The figure shows three views and two pictorial views of one solid part (mm, origin at its lowest corner). Answer the questions. Coordinates: 2 decimals unless noted, no trailing zeros. Order: outer loops, then holes, each group sorted by start corner. A loop starts at its lowest first (then second) coordinate and runs counter-clockwise, first axis right, second up. Notation, with made-up numbers: (-3.5, 69) -> (38.5, 69) arc R24 ccw to (38.5, 87) -> close; hole circle Ø4 at (-25.5, -30.5). An arc over 180 degrees is marked (long way). Write item = value, one per line.
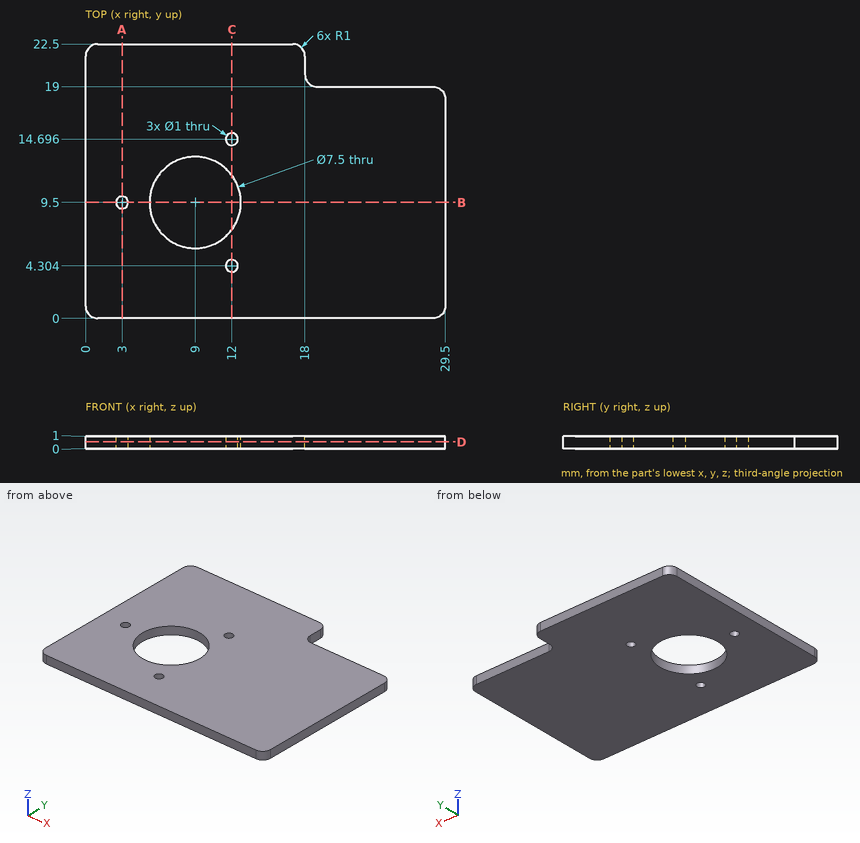
Q1. Section B-B, the plane y = 9.5 is taken. Give the vertices of the cut face in (x, z), plus the area to 3 significant figures.
The answers:
outline = (0, 0) -> (2.5, 0) -> (2.5, 1) -> (0, 1) -> close; (3.5, 0) -> (5.25, 0) -> (5.25, 1) -> (3.5, 1) -> close; (12.75, 0) -> (29.5, 0) -> (29.5, 1) -> (12.75, 1) -> close
area = 21.0 mm2
Q2. Section D-D, the plane z = 0.55 is taken. Give the vertices of the cut face in (x, y).
The answers:
outline = (0, 1) arc R1 ccw to (1, 0) -> (28.5, 0) arc R1 ccw to (29.5, 1) -> (29.5, 18) arc R1 ccw to (28.5, 19) -> (19, 19) arc R1 cw to (18, 20) -> (18, 21.5) arc R1 ccw to (17, 22.5) -> (1, 22.5) arc R1 ccw to (0, 21.5) -> close; hole circle Ø1 at (3, 9.5); hole circle Ø7.5 at (9, 9.5); hole circle Ø1 at (12, 4.3); hole circle Ø1 at (12, 14.7)
Q3. Section C-C, the plane x = 12 is taken. Give the vertices of the cut face in (y, z).
The answers:
outline = (0, 0) -> (3.8, 0) -> (3.8, 1) -> (0, 1) -> close; (4.8, 0) -> (7.25, 0) -> (7.25, 1) -> (4.8, 1) -> close; (11.75, 0) -> (14.2, 0) -> (14.2, 1) -> (11.75, 1) -> close; (15.2, 0) -> (22.5, 0) -> (22.5, 1) -> (15.2, 1) -> close
Q4. Find the intervals of material crossed by line 1 along Y through (x, z) = (12, 0.4); line 2 along Y through (x, z) = (9, 0.5); line 3 along Y through (x, z) = (24, 0.4), in increasing order.
The answers:
line_1 = 0 to 3.8, 4.8 to 7.25, 11.75 to 14.2, 15.2 to 22.5
line_2 = 0 to 5.75, 13.25 to 22.5
line_3 = 0 to 19
Q5. Section A-A, the plane x = 3 is taken. Give the vertices of the cut face in (y, z), plus the area to 3 significant figures.
The answers:
outline = (0, 0) -> (9, 0) -> (9, 1) -> (0, 1) -> close; (10, 0) -> (22.5, 0) -> (22.5, 1) -> (10, 1) -> close
area = 21.5 mm2
